Design review of the part shown in the three views and the two pictorial views. Dimensions are in mm from the part's minimum x, y and z. Coordinates: 2 decimals unless noted, no trailing zeros. Order: outer loops, then holes, each group sorted by start corner. A loop starts at its lowest first (then second) coordinate and runs counter-clockwise, first axis right, second up. Notation, with made-up numbers: (-10.75, -13) -> (29.25, -13) arc R12 cw to (29.25, 10) -> close; hole circle Ø6 at (37, 12.5). An arc over 180 degrees is marked (long way). Write item = value, one per line. Start each with the question number.
1) Wall thickness on probe 1 along Z at (x, y) = (58, 18) (1 decimal); probe 2 along Y at (x, z) = (242, 50); probe 3 along X at (y, z) = (31, 390.5): over which ranges is each line inside the solid? List them lowest first. Write a range as [from, to].
2) Consider section B-B on z = 400. Give the boundary of the cut face in (x, y), and give its area (3 significant figures).
3) Consider section A-A on y = 19. Give the boundary of the cut face in (x, z) (1 decimal).
4) Consider section D-D on x = 26. Give the boundary of the cut face in (y, z).
5) Consider section C-C on x = 66. Give the boundary of the cut face in (y, z) (1 decimal), and give its area (3 significant figures).
6) Insertion check: pin 1 Ø5 at (x, y) = (245.5, 4) entering from -Z; pin 2 Ø5 at (y, z) = (7, 240) entering from -X; pin 3 Ø2 at (x, z) = (102, 62.5) entering from -Y. Each pin has a flat end and moves straight along its axis. Give the tip position at first contact, or say it passes through.
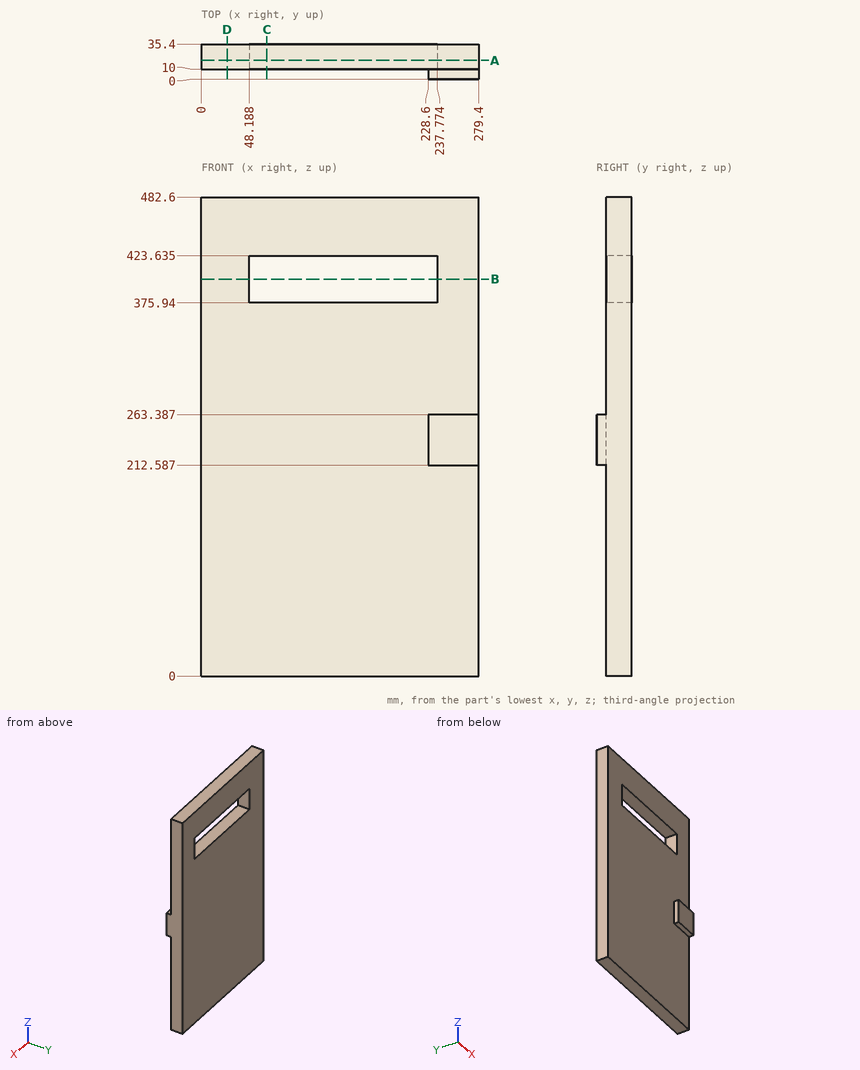
Answer sheet:
q1.probe_1 = [0, 375.9], [423.6, 482.6]
q1.probe_2 = [10, 35.4]
q1.probe_3 = [0, 48.19], [237.77, 279.4]
q2.outline = (0, 10) -> (48.19, 10) -> (48.19, 35.4) -> (0, 35.4) -> close; (237.77, 10) -> (279.4, 10) -> (279.4, 35.4) -> (237.77, 35.4) -> close
q2.area = 2,280 mm2
q3.outline = (0, 0) -> (279.4, 0) -> (279.4, 482.6) -> (0, 482.6) -> close; hole (48.2, 375.9) -> (237.8, 375.9) -> (237.8, 423.6) -> (48.2, 423.6) -> close
q4.outline = (10, 0) -> (35.4, 0) -> (35.4, 482.6) -> (10, 482.6) -> close
q5.outline = (10, 0) -> (35.4, 0) -> (35.4, 375.9) -> (10, 375.9) -> close; (10, 423.6) -> (35.4, 423.6) -> (35.4, 482.6) -> (10, 482.6) -> close
q5.area = 11,000 mm2
q6.pin_1 = 212.59
q6.pin_2 = 228.6
q6.pin_3 = 10
